```python
from build123d import *

# Parameters (mm, degrees)
BASE_FLANGE1_DEPTH = 150
SKETCH2_R          = 1.25
CUT_EXTRUDE1_DEPTH = 10


# Sheet-metal steps are written as plain solids
with BuildPart() as part:
    # Sketch1 → Base-Flange1 (new body)
    with BuildSketch(Plane(origin=(0, 0, 0), x_dir=(0, 0, -1), z_dir=(1, 0, 0))):
        with BuildLine():
            Line((0, 0), (0, 7.5))
            ThreePointArc((0, 7.5), (-0.146446609, 7.853553391), (-0.5, 8))
            Line((-0.5, 8), (-78.5, 8))
            ThreePointArc((-78.5, 8), (-79.560660172, 8.439339828), (-80, 9.5))
            Line((-80, 9.5), (-80, 13))
            Line((-80, 13), (-79, 13))
            Line((-79, 13), (-79, 9.5))
            ThreePointArc((-79, 9.5), (-78.853553391, 9.146446609), (-78.5, 9))
            Line((-78.5, 9), (-0.5, 9))
            ThreePointArc((-0.5, 9), (0.560660172, 8.560660172), (1, 7.5))
            Line((1, 7.5), (1, 0))
            Line((1, 0), (0, 0))
        make_face()
    extrude(amount=BASE_FLANGE1_DEPTH)

    # Sketch2 → Cut-Extrude1 (cut)
    with BuildSketch(Plane(origin=(0, 0, -1), x_dir=(-1, 0, 0), z_dir=(0, 0, -1))):
        with Locations((-25, 3.75)):
            Circle(SKETCH2_R)
        with Locations((-125, 3.75)):
            Circle(SKETCH2_R)
    extrude(amount=-CUT_EXTRUDE1_DEPTH, mode=Mode.SUBTRACT)


solid = part.part
```
Geometry: final body of the model. Coordinates: model frame, mm. A direction names the side the tool comes from. Give positions to 0.01 mm unless a question says otherwise; leave off trailing zeros. Loops run counter-clockwise (first coordinate to the right, second up) from the corner with the lowest first, then second, coordinate; pieces in that order, holes last. Notation, with made-up numbers: (46, 4) -> (103, 4) arc R12 cw to (103, 25) -> close; hole circle Ø11 at (-27.5, -1). An arc over 180 degrees is marked (long way). Use one line per item in the form item = value.
Item 1: Section query B-B on z = 20.5. Output: boundary loops of the cut face in (x, y).
A:
outline = (0, 8) -> (150, 8) -> (150, 9) -> (0, 9) -> close
Item 2: Section query A-A on x = 88.5. Output: boundary loops of the cut face in (y, z).
A:
outline = (0, -1) -> (7.5, -1) arc R1.5 ccw to (9, 0.5) -> (9, 78.5) arc R0.5 cw to (9.5, 79) -> (13, 79) -> (13, 80) -> (9.5, 80) arc R1.5 ccw to (8, 78.5) -> (8, 0.5) arc R0.5 cw to (7.5, 0) -> (0, 0) -> close
Item 3: Pin query (flat end, axial travel): P1, Ø4, axis at x = 130, z = 46, coming from the +Y side; P2, Ø1, axis at x = 66, z = 21.5, coming from the -Y side; P3, Ø3, axis at x = 107.5, y = 11.5, coming from the -Z side. Return the tip coordinate at first contact, or that it passes through.
A:
P1 = 9
P2 = 8
P3 = 79
Item 4: Access query for faces 1 (the face through (74, 11, 79)), 2 (the face through (150, 8.5, 39.3)), 3 (the face through (74, 4, 0)). Directions: +Z, -Z, +X, -X, +Y, -Y. A direction counts if a zero-diameter tool reaches every point of the face in a straight line with its end or side. Return the directions, or none.
A:
face_1 = -Z, +X, -X, +Y
face_2 = +Z, -Z, +X, +Y, -Y
face_3 = +Z, +X, -X, -Y
Item 5: Line query: probe 1 along Y at (x, z) = (56, 46); probe 2 along Z at (x, y) = (29, 10); probe 3 along Z at (x, y) = (46, 2.75). Output: solid intervals per line, ascending.
A:
probe_1 = 8 to 9
probe_2 = 79 to 80
probe_3 = -1 to 0
